Source: CAD feature listing. Evaluate the final solid. Frame: model axes, mm. A direction names the side the tool comes from. Coordinates: 2 decimals unless noted, no trailing zeros. Order: outer loops, then holes, each group sorted by start corner. A loop starts at its lowest first (then second) coordinate and runs counter-clockwise, first axis right, second up.
Item 1: Section D-D on z = 13.5. Return the cut outline in (x, y), then the cut area to 3 significant figures.
Item 2: Section C-C on y = 5.5. Return the cut outline in (x, z).
Item 3: Ray query, line 1 (X direction, y = 6, z = 0); line 2 (X direction, y = 0.65, z = 0); line 3 (Y direction, x = 1, z = 12). Return the intervals inside material, ascending.
Item 4: Reachability of faces 5 (the flat face through (-12.15, 2, 1.15)), 6 (the cylindrical face through (-16.108, 0.986, -3.577)) from +Z, -Z, +X, -X, +Y, -Y: full face, straight path, thin tool, end or side. Return the list, or none.
Item 5: Mould query, pull axis Z, two halves, no side actions, for faces 1 (the cylindrical face through (3.604, 7.423, 11.446)), 2 (the cylindrical face through (2.703, 0.493, -8.584)), 3 (the flat face through (-7, 0, 7)), 4 (the flat face through (7.4, 1, 2)). Classes: released by +Z, released by -Z, zero draft, split by the parting line, or undercut.
Item 6: Section A-A on x = 0. Return the cut outline in (y, z), then the cut area to 3 significant figures.
Item 7: Section B-B on z = 0. Return the cut outline in (x, y), then the cut area to 3 significant figures.
Item 8: Contact query for a flat-ended pin moving along its axis: P1, Ø5, axis at y = 3.5, z = 2.5, coming from the -X side. Output: stop coordinate, or through.
from build123d import *

# Parameters (mm, degrees)
SKETCH1_R           = 16.5
BOSS_EXTRUDE1_DEPTH = 2
SKETCH2_R           = 12
BOSS_EXTRUDE2_DEPTH = 11
SKETCH3_R           = 9
CUT_EXTRUDE1_DEPTH  = 1
SKETCH4_R           = 7.5
CUT_EXTRUDE2_DEPTH  = 12


with BuildPart() as part:
    # Sketch1 → Boss-Extrude1 (new body)
    with BuildSketch(Plane(origin=(0, 0, 0), x_dir=(1, 0, 0), z_dir=(0, 1, 0))):
        with Locations(Location((0, 0, 0), (0, 0, 270))):
            Circle(SKETCH1_R)
    extrude(amount=BOSS_EXTRUDE1_DEPTH)

    # Sketch2 → Boss-Extrude2 (add)
    with BuildSketch(Plane(origin=(0, 2, 0), x_dir=(1, 0, 0), z_dir=(0, 1, 0))):
        with Locations(Location((0, 0, 0), (0, 0, 270))):
            Circle(SKETCH2_R)
    extrude(amount=BOSS_EXTRUDE2_DEPTH)

    # Sketch3 → Cut-Extrude1 (cut)
    with BuildSketch(Plane.XZ):
        with Locations(Location((0, 0, 0), (0, 0, 270))):
            Circle(SKETCH3_R)
    extrude(amount=-CUT_EXTRUDE1_DEPTH, mode=Mode.SUBTRACT)

    # Sketch4 → Cut-Extrude2 (cut)
    with BuildSketch(Plane(origin=(0, 13, 0), x_dir=(1, 0, 0), z_dir=(0, 1, 0))):
        with Locations(Location((0, 0, 0), (0, 0, 270))):
            Circle(SKETCH4_R)
    extrude(amount=-CUT_EXTRUDE2_DEPTH, mode=Mode.SUBTRACT)


solid = part.part
Answer list:
1. outline: (-9.49, 0) - (9.49, 0) - (9.49, 2) - (-9.49, 2) - close
1. area: 37.9 mm2
2. outline: circle Ø24 at (0, 0); hole circle Ø15 at (0, 0)
3. line 1: x = -12 to -7.5, 7.5 to 12
3. line 2: x = -16.5 to -9, 9 to 16.5
3. line 3: y = 0 to 2
4. face 5: +Y
4. face 6: +Y, -Y
5. face 1: split by the parting line
5. face 2: undercut
5. face 3: zero draft
5. face 4: undercut
6. outline: (0, -16.5) - (2, -16.5) - (2, -12) - (13, -12) - (13, -7.5) - (1, -7.5) - (1, -9) - (0, -9) - close; (0, 9) - (1, 9) - (1, 7.5) - (13, 7.5) - (13, 12) - (2, 12) - (2, 16.5) - (0, 16.5) - close
6. area: 132 mm2
7. outline: (-16.5, 0) - (-9, 0) - (-9, 1) - (-7.5, 1) - (-7.5, 13) - (-12, 13) - (-12, 2) - (-16.5, 2) - close; (7.5, 1) - (9, 1) - (9, 0) - (16.5, 0) - (16.5, 2) - (12, 2) - (12, 13) - (7.5, 13) - close
7. area: 132 mm2
8. P1: stops at x = -16.49
